Can you work these out from the model? Positions are in its coordinate system, mm. A direction names the side the tool comes from. Give positions to 0.01 mm unless a question says otherwise; leave off trailing zeros. Order: outer loops, then holes, each group sorted by start corner. A loop starts at its lowest first (then second) coordinate and runs counter-clockwise, first axis right, second up. Notation, with made-up numbers: M 40,-7 L 73,-7 A11 cw 73,7 Z; hole C 4,-34.75 d5. An arc over 180 degrees is marked long. Answer as a JSON object with one key per item and string values.
```python
from build123d import *

# Parameters (mm, degrees)
F0_R     = 8.89
F1_DEPTH = 50
F3_DEPTH = 50
F4_DEPTH = 80


with BuildPart() as f1:
    # F0 (on Right) → F1 (new body)
    with BuildSketch(Plane.YZ):
        Polygon((-101.6, -50.8), (72.478287, -50.8), (101.6, -13.316209), (49.016677, 50.8), (-101.6, 50.8), align=None)
        with Locations((-54.578975, -38.1)):
            Circle(F0_R, mode=Mode.SUBTRACT)
        with Locations((50.709363, -38.1)):
            Circle(F0_R, mode=Mode.SUBTRACT)
    extrude(amount=F1_DEPTH)

    # F2 (on face) → F3 (cut)
    with BuildSketch(Plane.YZ.offset(50)):
        Polygon((-101.6, 50.8), (-101.6, 16.903477), (76.816072, 16.903477), (49.016677, 50.8), align=None)
    extrude(amount=-F3_DEPTH, mode=Mode.SUBTRACT)

    # F0 (on Right) → F4 (join)
    with BuildSketch(Plane.YZ):
        with Locations((50.709363, -38.1)):
            Circle(F0_R)
    extrude(amount=F4_DEPTH)

    # F5: F1 across plane


with BuildPart() as f1_1:
    add(f1.part)
    add(f1.part.mirror(Plane.YZ))


solid = f1_1.part
```
1) I want a section at D-D on z = 1.5. Write out the boundary of the cut face in (x, y).
Results found:
{"outline": "M -50,-101.6 L 50,-101.6 L 50,89.45 L -50,89.45 Z"}
2) I want a section at C-C on y = 53. Write out the boundary of the cut face in (x, z).
Results found:
{"outline": "M -80,-46.69 L -50,-46.69 L -50,-50.8 L 50,-50.8 L 50,-46.69 L 80,-46.69 L 80,-29.51 L 50,-29.51 L 50,16.9 L -50,16.9 L -50,-29.51 L -80,-29.51 Z"}
3) I want a section at A-A on x = -30.5. Write out the boundary of the cut face in (y, z).
Results found:
{"outline": "M -101.6,-50.8 L 72.48,-50.8 L 101.6,-13.32 L 76.82,16.9 L -101.6,16.9 Z; hole C -54.58,-38.1 d17.78"}
4) For faces 1 (the face through (1, -16, -50.8)), 2 (the face through (64.79, 58.921, -41.505)), 3 (the face through (-64.79, 58.921, -41.505)), which set-ups out of +Z, -Z, +X, -X, +Y, -Y let a thin tool reach every point of the face, with its end or its side?
Results found:
{"face 1": "-Z, +X, -X, +Y, -Y", "face 2": "+X", "face 3": "-X"}
5) I need wall thicknesses on L1, parallel to X at y = -58.5, z = 3; L2, parallel to Y at x = -31, z = -38; L3, parallel to Y at x = 13.5, z = -38.5. Which ranges of each line are inside material? Lowest first, please.
Results found:
{"L1": "x = -50 to 50", "L2": "y = -101.6 to -63.47, -45.69 to 82.42", "L3": "y = -101.6 to -63.46, -45.7 to 82.03"}
6) I want a section at B-B on z = -38.1. Write out the boundary of the cut face in (x, y), and give its area (3 significant figures).
Results found:
{"outline": "M -80,41.82 L -50,41.82 L -50,-45.69 L 50,-45.69 L 50,41.82 L 80,41.82 L 80,59.6 L 50,59.6 L 50,82.35 L -50,82.35 L -50,59.6 L -80,59.6 Z; M -50,-101.6 L 50,-101.6 L 50,-63.47 L -50,-63.47 Z", "area": "17,700 mm²"}
7) I'm going to push flat-ended pins straight in: pin 1 Ø1.5 at (y, z) = (-26.5, -10) entering from -X; pin 2 Ø1.5 at (x, z) = (26, 6.5) entering from +Y; pin 3 Ø10.5 at (y, z) = (-54.58, -38.1) entering from -X; pin 4 Ø20.5 at (y, z) = (23, -12.5) entering from +X. Where does each tip first touch, or does it pass through?
Results found:
{"pin 1": "stops at x = -50", "pin 2": "stops at y = 85.96", "pin 3": "passes through", "pin 4": "stops at x = 50"}
